```python
from build123d import *

# Parameters (mm, degrees)
SKETCH1_R           = 0.85
BOSS_EXTRUDE1_DEPTH = 1.4
SKETCH2_R           = 2.5
SKETCH2_R_2         = 0.85
BOSS_EXTRUDE2_DEPTH = 1
SKETCH3_R           = 1
CUT_EXTRUDE1_DEPTH  = 0.1


with BuildPart() as part:
    # Sketch1 → Boss-Extrude1 (new body)
    with BuildSketch(Plane.XY):
        with BuildLine():
            Line((-5.340410415, 0.85), (-5.93948651, 0.85))
            ThreePointArc((-5.93948651, 0.85), (-5.071934946, 3.205538317), (-3.31662479, 5))
            Line((-3.31662479, 5), (3.31662479, 5))
            ThreePointArc((3.31662479, 5), (5.071934946, 3.205538317), (5.93948651, 0.85))
            Line((5.93948651, 0.85), (5.340410415, 0.85))
            Line((5.340410415, 0.85), (5.340410415, -0.85))
            Line((5.340410415, -0.85), (5.93948651, -0.85))
            ThreePointArc((5.93948651, -0.85), (5.071934946, -3.205538317), (3.31662479, -5))
            Line((3.31662479, -5), (-3.31662479, -5))
            ThreePointArc((-3.31662479, -5), (-5.071934946, -3.205538317), (-5.93948651, -0.85))
            Line((-5.93948651, -0.85), (-5.340410415, -0.85))
            Line((-5.340410415, -0.85), (-5.340410415, 0.85))
        make_face()
        Circle(SKETCH1_R, mode=Mode.SUBTRACT)
    extrude(amount=BOSS_EXTRUDE1_DEPTH)

    # Sketch2 → Boss-Extrude2 (add)
    with BuildSketch(Plane.XY.offset(1.4)):
        Circle(SKETCH2_R)
        Circle(SKETCH2_R_2, mode=Mode.SUBTRACT)
    extrude(amount=BOSS_EXTRUDE2_DEPTH)

    # Sketch3 → Cut-Extrude1 (cut)
    # profile 1 of 3: a face of its own
    with BuildSketch(Plane.XY.offset(1.4)):
        with Locations((0, 3.75)):
            Circle(SKETCH3_R)
    # profile 2 of 3: a face of its own
    with BuildSketch(Plane.XY.offset(1.4)):
        with Locations((-3.006653395, -2.766898706)):
            Circle(SKETCH3_R)
    # profile 3 of 3: a face of its own
    with BuildSketch(Plane.XY.offset(1.4)):
        with Locations(Location((3.006653395, -2.766898706, 0), (0, 0, 180))):
            Circle(SKETCH3_R)
        Polygon((3.166281654, -2.605998411), (3.930459475, -2.605998411), (3.930459475, -2.927799001), (3.166281654, -2.927799001), (3.166281654, -3.683401413), (2.847025136, -3.683401413), (2.847025136, -2.927799001), (2.082847315, -2.927799001), (2.082847315, -2.605998411), (2.847025136, -2.605998411), (2.847025136, -1.850395999), (3.166281654, -1.850395999), align=None, mode=Mode.SUBTRACT)
    extrude(amount=-CUT_EXTRUDE1_DEPTH, mode=Mode.SUBTRACT)


solid = part.part
```
Work out the finished part from the listing and answer in its coordinate system (mm). A direction names the side the tool comes from. Round coordinates to 2 decimals unless told otherwise and drop trailing zeros. Write each loop counter-clockwise with the first axis right and the second up, starting at its lowest first coordinate (ties: lowest second). Pieces come first, ordered by that corner, then holes. Notation, with made-up numbers: (83, 48) - (110, 48) arc R20 cw to (110, 65) - close; hole circle Ø5 at (6, -18). An arc over 180 degrees is marked (long way). Return JSON: item names as keys, results as strings. Group by question number.
Q1. The mould has two halves that part along Y. Classify faces 4 (the flat face through (0, 5, 1)), 5 (the flat face through (0, 4, 1.3)), 6 (the flat face through (0, -5, 1)): released by +Y, released by -Y, zero draft, split by the parting line, or undercut.
Q2. Each of these flat-tipped pins is pushed along its axis until it touches: pin 1 Ø3 at (x, y) = (4.5, -3.5) entering from +Z; pin 2 Ø6 at (x, y) = (1.5, -1) entering from -Z. Where does it stop, or does it pass through?
Q3. For faces 1 (the flat face through (-3, -3, 1.3)), 2 (the flat face through (5.34, 0, 1)), 3 (the flat face through (-5.34, 0, 1)), determine the directions among +Z, -Z, +X, -X, +Y, -Y from which every point of the face is accessible in a straight line to the end or side of a thin tool.
Q4. The part is cut by section A-A on y = 0. Write down the section's boundary in (x, z).
Q5. Find the intervals of material crossed by L1, parallel to Y at x = 0, z = 1.35; L2, parallel to Y at x = 0, z = 1.2; L3, parallel to Z at x = 4, y = -4.25, in increasing order.
Q6. The part is cut by section C-C on z = 0.5. Write down the section's boundary in (x, y).
Q7. The part is cut by section D-D on y = 3.75. Write down the section's boundary in (x, z), then the cut area to 3 significant figures.
Q8. The part is cut by section B-B on x = 0. Write down the section's boundary in (y, z), then the cut area to 3 significant figures.
Solved:
{
 "1": {"face 4": "released by +Y", "face 5": "undercut", "face 6": "released by -Y"},
 "2": {"pin 1": "z = 1.4", "pin 2": "z = 0"},
 "3": {"face 1": "+Z", "face 2": "+Z, -Z, +X", "face 3": "+Z, -Z, -X"},
 "4": {"outline": "(-5.34, 0) - (-0.85, 0) - (-0.85, 2.4) - (-2.5, 2.4) - (-2.5, 1.4) - (-5.34, 1.4) - close; (0.85, 0) - (5.34, 0) - (5.34, 1.4) - (2.5, 1.4) - (2.5, 2.4) - (0.85, 2.4) - close"},
 "5": {"L1": "-5 to -0.85, 0.85 to 2.75, 4.75 to 5", "L2": "-5 to -0.85, 0.85 to 5", "L3": "0 to 1.4"},
 "6": {"outline": "(-5.94, -0.85) arc R6 ccw to (-3.32, -5) - (3.32, -5) arc R6 ccw to (5.94, -0.85) - (5.34, -0.85) - (5.34, 0.85) - (5.94, 0.85) arc R6 ccw to (3.32, 5) - (-3.32, 5) arc R6 ccw to (-5.94, 0.85) - (-5.34, 0.85) - (-5.34, -0.85) - close; hole circle Ø1.7 at (0, 0)"},
 "7": {"outline": "(-4.68, 0) - (4.68, 0) - (4.68, 1.4) - (1, 1.4) - (1, 1.3) - (-1, 1.3) - (-1, 1.4) - (-4.68, 1.4) - close", "area": "12.9 mm²"},
 "8": {"outline": "(-5, 0) - (-0.85, 0) - (-0.85, 2.4) - (-2.5, 2.4) - (-2.5, 1.4) - (-5, 1.4) - close; (0.85, 0) - (5, 0) - (5, 1.4) - (4.75, 1.4) - (4.75, 1.3) - (2.75, 1.3) - (2.75, 1.4) - (2.5, 1.4) - (2.5, 2.4) - (0.85, 2.4) - close", "area": "14.7 mm²"}
}
